Input: dimensioned drawing with shaded views. Units: mm. Origin: part minimum x, y, z. Round coordinates to 2 decimals unless told otherwise and drop trailing zeros. Write each loop counter-clockwise with the first axis right and the second up, starting at its lowest first coordinate (ties: lowest second). Pieces come first, ordered by that corner, then holes. Notation, with made-up numbers: (71.5, -12.5) -> (79.5, -12.5) arc R5 ccw to (79.5, -7.5) -> close; hole circle Ø11 at (0, 19). An arc over 180 degrees is marked (long way). Use one line per item in the form item = value. Start each with the question number.
1. Pin query (flat end, axial travel): pin 1 Ø1 at (x, y) = (11, 8) entering from +Z; pin 2 Ø1.5 at (x, z) = (7, 33) entering from +Y; pin 3 Ø1.5 at (x, y) = (8, 9) entering from -Z. Return the tip coordinate at first contact, or that it passes through.
2. Line query: L1, parallel to Z at x = 8.5, y = 3.5; L2, parallel to Z at x = 7.5, y = 5.75; L3, parallel to Z at x = 8, y = 1.25. Output: solid intervals per line, ascending.
3. Draft query along X for the marked faces 1, 2 and 3. Return one class per face: pulls with the +X half, pulls with the -X half, needs draft (parallel to the pull), parting line crosses it, or undercut.
4. Cut plane D-D, the plane y = 3.5. Return the cut outline in (x, z) (3 decimals), plus the area to 3 significant figures.
5. Cut plane B-B, the plane z = 24.5. Return the cut outline in (x, y), plus the area to 3 significant figures.
6. Cut plane C-C, the plane y = 9. Return the cut outline in (x, z), plus the area to 3 significant figures.
7. Cut plane A-A, the plane x = 8.5. Return the cut outline in (y, z), plus the area to 3 significant figures.
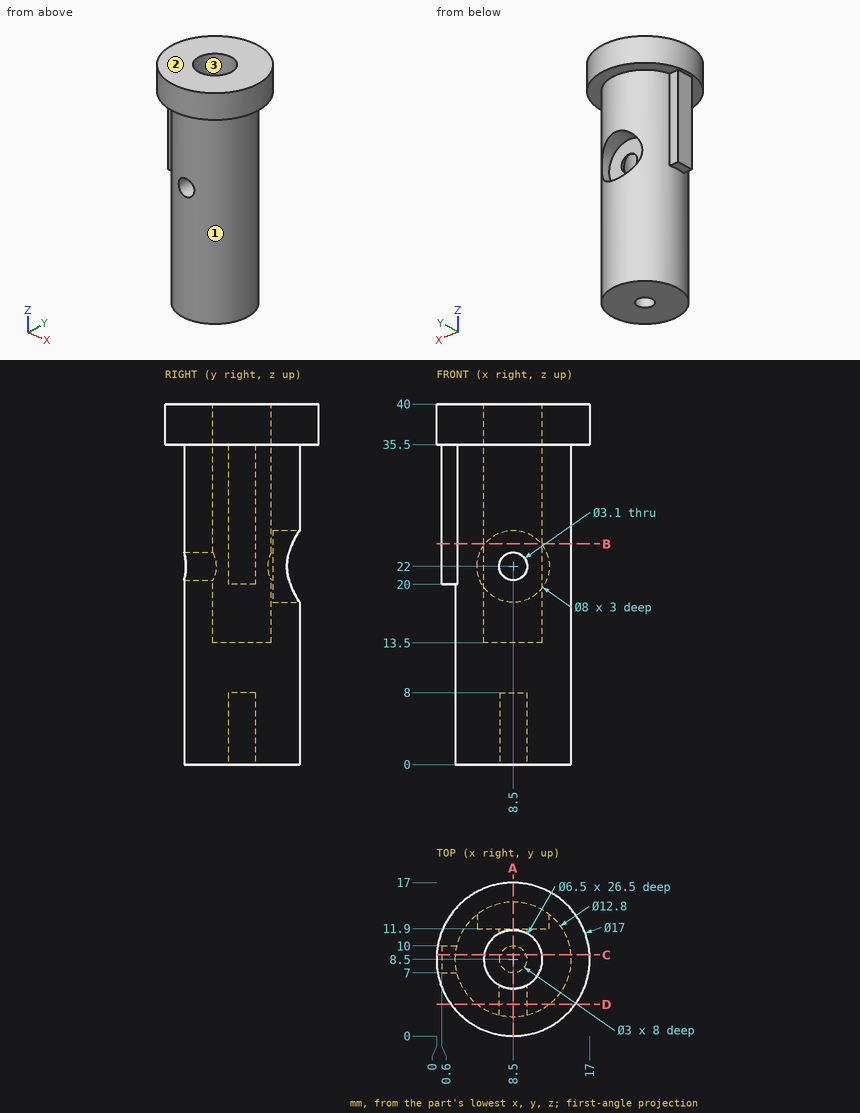
Outcome:
q1.pin_1 = 13.5
q1.pin_2 = 14.86
q1.pin_3 = 8
q2.L1 = 0 to 20.45, 23.55 to 40
q2.L2 = 0 to 13.5
q2.L3 = 35.5 to 40
q3.face_1 = parting line crosses it
q3.face_2 = needs draft
q3.face_3 = undercut
q4.outline = (1.626, 35.5) -> (4.505, 35.5) -> (4.505, 0) -> (12.495, 0) -> (12.495, 35.5) -> (15.374, 35.5) -> (15.374, 40) -> (1.626, 40) -> close; hole circle Ø3.1 at (8.5, 22)
q4.area = 338 mm^2
q5.outline = (0.6, 7) -> (2.28, 7) arc R6.4 ccw (long way) to (11.62, 14.09) -> (11.62, 11.9) -> (5.38, 11.9) -> (5.38, 14.09) arc R6.4 ccw to (2.28, 10) -> (0.6, 10) -> close; hole circle Ø6.5 at (8.5, 8.5)
q5.area = 83.1 mm^2
q6.outline = (0.01, 35.5) -> (0.6, 35.5) -> (0.6, 20) -> (2.12, 20) -> (2.12, 0) -> (7.09, 0) -> (7.09, 8) -> (9.91, 8) -> (9.91, 0) -> (14.88, 0) -> (14.88, 35.5) -> (16.99, 35.5) -> (16.99, 40) -> (11.71, 40) -> (11.71, 13.5) -> (5.29, 13.5) -> (5.29, 40) -> (0.01, 40) -> close
q6.area = 360 mm^2
q7.outline = (0, 35.5) -> (2.1, 35.5) -> (2.1, 23.55) -> (5.25, 23.55) -> (5.25, 40) -> (0, 40) -> close; (2.1, 0) -> (7, 0) -> (7, 8) -> (10, 8) -> (10, 0) -> (14.9, 0) -> (14.9, 18) -> (11.9, 18) -> (11.9, 20.45) -> (11.75, 20.45) -> (11.75, 13.5) -> (5.25, 13.5) -> (5.25, 20.45) -> (2.1, 20.45) -> close; (11.75, 23.55) -> (11.9, 23.55) -> (11.9, 26) -> (14.9, 26) -> (14.9, 35.5) -> (17, 35.5) -> (17, 40) -> (11.75, 40) -> close
q7.area = 300 mm^2
